Can you work these out from the model? Positions are in its coordinate system, mm. A direction names the side the tool comes from. Coordinates: 2 decimals unless noted, no trailing zeros. Order: outer loops, then holes, each group sorted by start corner. A loop starts at its lowest first (then second) coordinate and runs counter-clockwise, first axis right, second up. Notation, with made-up numbers: (66, 25) -> (88, 25) arc R14 ccw to (88, 34) -> close; hole circle Ø11 at (-24, 15.25). An arc over 180 degrees is marked (long way). Answer in a Markdown table with one row per item. Add a question column.
1. Will these pins go through, and if not, where does the flat tip stop? pin 1 (4 mm diameter, centred on x = 10, y = 11.5, fed in from -Z); pin 2 (4 mm diameter, centred on y = 1.5, z = -14, fed in from -X); pin 3 (2 mm diameter, centred on y = 14.5, z = 17.5, fed in from +X).
2. Imagine slicing it at C-C on y = 7.5. Write out the boundary of the cut face in (x, z), plus the area to 3 significant figures.
3. Imagine slicing it at B-B on x = 2. Write out the boundary of the cut face in (y, z).
4. If I drill on line 1 along X through (y, z) = (7, 0); line 2 along Y through (x, z) = (1.5, 17); line 3 along X through (y, z) = (8.5, 2), over which ranges is the centre line in solid material (lowest first)? Write a range as [from, to].
5. On a 3-axis mill with a long thin cutter (end or side, diameter ignored), from which of +Z, -Z, +X, -X, +Y, -Y can I reach the whole of each face in a straight line? I mean faces 1 (the face through (-19.83, 12.53, -2.6)), 2 (the face through (0, 14, -16)), 3 (the face through (10.5, 11, 10.3)). Say none if no direction works.
6. Imagine slicing it at A-A on z = 0. Write out the boundary of the cut face in (x, y), plus the area to 3 significant figures.
7. Imagine slicing it at D-D on z = 17. Write out the boundary of the cut face in (x, y), plus the area to 3 significant figures.
from build123d import *

# Parameters (mm, degrees)
SKETCH_2_R      = 14.5
SKETCH_2_R_2    = 12.5
EXTRUDE_1_DEPTH = 11
SKETCH_3_R      = 20
SKETCH_3_R_2    = 12.5
EXTRUDE_2_DEPTH = 2
EXTRUDE_3_DEPTH = 2


with BuildPart() as part:
    # 草圖2 → 填料-伸長1 (new body)
    with BuildSketch(Plane(origin=(0, 0, 0), x_dir=(1, 0, 0), z_dir=(0, 1, 0))):
        with Locations(Location((0, 0, 0), (0, 0, 270))):
            Circle(SKETCH_2_R)
        with Locations(Location((0, 0, 0), (0, 0, 270))):
            Circle(SKETCH_2_R_2, mode=Mode.SUBTRACT)
    extrude(amount=EXTRUDE_1_DEPTH)

    # 草圖3 → 填料-伸長2 (add)
    with BuildSketch(Plane(origin=(0, 11, 0), x_dir=(1, 0, 0), z_dir=(0, 1, 0))):
        with Locations(Location((0, 0, 0), (0, 0, 270))):
            Circle(SKETCH_3_R)
        with Locations(Location((0, 0, 0), (0, 0, 270))):
            Circle(SKETCH_3_R_2, mode=Mode.SUBTRACT)
    extrude(amount=EXTRUDE_2_DEPTH)

    # 草圖4 → 填料-伸長3 (add)
    with BuildSketch(Plane(origin=(0, 13, 0), x_dir=(1, 0, 0), z_dir=(0, 1, 0))):
        with BuildLine():
            Line((0, 20), (0, 12.5))
            ThreePointArc((0, 12.5), (-12.5, 0), (0, -12.5))
            Line((0, -12.5), (0, -20))
            ThreePointArc((0, -20), (-20, 0), (0, 20))
        make_face()
    extrude(amount=EXTRUDE_3_DEPTH)


solid = part.part
Answers follow:
| question | item | result |
|---|---|---|
| 1 | pin 1 | stops at z = -18.33 |
| 1 | pin 2 | stops at x = -8.14 |
| 1 | pin 3 | stops at x = 0 |
| 2 | outline | circle Ø29 at (0, 0); hole circle Ø25 at (0, 0) |
| 2 | area | 170 mm² |
| 3 | outline | (0, -14.36) -> (11, -14.36) -> (11, -19.9) -> (13, -19.9) -> (13, -12.34) -> (0, -12.34) -> close; (0, 12.34) -> (13, 12.34) -> (13, 19.9) -> (11, 19.9) -> (11, 14.36) -> (0, 14.36) -> close |
| 4 | line 1 | x = [-14.5, -12.5], [12.5, 14.5] |
| 4 | line 2 | y = [11, 13] |
| 4 | line 3 | x = [-14.36, -12.34], [12.34, 14.36] |
| 5 | face 1 | +Y, -Y |
| 5 | face 2 | +Z, -Z, +X, +Y |
| 5 | face 3 | -Y |
| 6 | outline | (-20, 11) -> (-14.5, 11) -> (-14.5, 0) -> (-12.5, 0) -> (-12.5, 15) -> (-20, 15) -> close; (12.5, 0) -> (14.5, 0) -> (14.5, 11) -> (20, 11) -> (20, 13) -> (12.5, 13) -> close |
| 6 | area | 89.0 mm² |
| 7 | outline | (-10.54, 11) -> (10.54, 11) -> (10.54, 13) -> (0, 13) -> (0, 15) -> (-10.54, 15) -> close |
| 7 | area | 63.2 mm² |
